Could you check a few things on this model? Use its own coordinates, in mm. A direction names the side the tool comes from. Coordinates: 2 decimals unless noted, no trailing zeros. Loops run counter-clockwise (first coordinate to the right, second up) from the corner with the lowest first, then second, coordinate; pieces in that order, holes last. Notation, with made-up numbers: (78.5, 44.5) -> (121.5, 44.5) arc R8 ccw to (121.5, 51.5) -> close; hole circle Ø5 at (58.25, -30.75). An arc over 180 degrees is marked (long way). One line per question, with ' | ' between items. Start each with the question number.
(1) I'm going to push flat-ended pins straight in: pin 1 Ø6 at (x, y) = (-2, 3.5) entering from -Z; pin 2 Ø1 at (x, y) = (-1, 11.5) entering from -Z; pin 3 Ø4 at (y, z) = (-2.5, -2) entering from -X. Where does each tip first touch, or does it pass through?
(2) Suppose I cut it at C-C (z = 0). Give the number of separate pieces and of enclosed holes in the cut face, plus the area to 3 significant figures.
(3) If we mould it in two halves opening along X, with no side actions, what happens to faces 1 (the face through (-2.3, -6, 0)), 2 (the face through (2.5, -3, 0)), 3 (the face through (0, 0, 0)), 4 (the face through (2.1, -3, 0))? For each: pulls with the +X half, pulls with the -X half, needs draft (parallel to the pull), parting line crosses it, or undercut.
(4) If I drill on line 1 along X through (y, z) = (-0.5, 1); line 2 along X through (y, z) = (6, 0); line 3 along Y through (x, z) = (2.4, 0), over which ranges is the centre line in solid material (lowest first)?
(5) Suppose I cut it at A-A (y = -4.7). Please give me the cut outline in (x, z).
(6) Suppose I cut it at B-B (y = 15.5). Please give me the cut outline in (x, z).
(7) Which directions (+Z, -Z, +X, -X, +Y, -Y) give clear straight access to the entire face, cutting with the end or side of a thin tool? Please do faces 5 (the face through (-2.5, -3, 0)), 6 (the face through (-1.049, 11.693, 4.725)), 7 (the face through (-2.303, -5.268, 0.295)), 8 (the face through (-2.1, -3, 0)).
```python
from build123d import *

# Parameters (mm, degrees)
CONG_1_R                = 0.2
CONG_2_R                = 0.2
CHANFREIN1_SIZE         = 0.7
CHANFREIN1_SIZE2        = 0.454585315
CONG_3_R                = 2
ESQUISSE2_W             = 0.4
ESQUISSE2_H             = 2.6
BOSS_EXTRU_1_DEPTH      = 6
ESQUISSE3_R             = 0.64
ENL_V_MAT_EXTRU_1_DEPTH = 6
CONG_4_R                = 1


with BuildPart() as part:
    # Esquisse1 → Révolution1 (revolve)
    with BuildSketch(Plane.XY):
        with BuildLine():
            Line((0, 18.8), (0, 0))
            Line((0, 0), (3.69, 0))
            Line((3.69, 0), (3.69, 7))
            Line((3.69, 7), (4.84, 7))
            Line((4.84, 7), (4.84, 15))
            Line((4.84, 15), (6.01, 15))
            Line((6.01, 15), (6.01, 16))
            ThreePointArc((6.01, 16), (5.013982948, 16.330092875), (4, 16.6))
            Line((4, 16.6), (4, 15.013190638))
            Line((4, 15.013190638), (3.89, 15.013190638))
            Line((3.89, 15.013190638), (3.89, 18.2))
            ThreePointArc((3.89, 18.2), (1.968000254, 18.649118314), (0, 18.8))
        make_face()
    revolve(axis=Axis((0, 0, 0), (0, 1, 0)))

    # Congé1
    cong_1_edges = [part.edges().sort_by_distance(p)[0] for p in [
        (-3.89, 18.2, 0),
    ]]
    fillet(cong_1_edges, radius=CONG_1_R)

    # Congé2
    cong_2_edges = [part.edges().sort_by_distance(p)[0] for p in [
        (-6.01, 16, 0),
    ]]
    fillet(cong_2_edges, radius=CONG_2_R)

    # Chanfrein1
    chanfrein1_edges = [part.edges().sort_by_distance(p)[0] for p in [
        (-4.84, 7, 0),
    ]]
    chanfrein1_side = [part.faces().sort_by_distance(p)[0] for p in [
        (-4.84, 11, 0),
    ]]
    chamfer(chanfrein1_edges, length=CHANFREIN1_SIZE, length2=CHANFREIN1_SIZE2, reference=chanfrein1_side[0])

    # Congé3
    cong_3_edges = [part.edges().sort_by_distance(p)[0] for p in [
        (-4.84, 7.7, 0),
    ]]
    fillet(cong_3_edges, radius=CONG_3_R)

    # Esquisse2 → Boss.-Extru.1 (add)
    with BuildSketch(Plane.XZ):
        with Locations((2.3, 0)):
            Rectangle(ESQUISSE2_W, ESQUISSE2_H)
        with Locations((-2.3, 0)):
            Rectangle(ESQUISSE2_W, ESQUISSE2_H)
    extrude(amount=BOSS_EXTRU_1_DEPTH)

    # Esquisse3 → Enlèv. mat.-Extru.1 (cut)
    with BuildSketch(Plane.ZY.offset(2.5)):
        with Locations((0, -4.7)):
            Circle(ESQUISSE3_R)
        with BuildLine():
            Line((-1.3, -0.8), (-4.192462756, -0.8))
            Line((-4.192462756, -0.8), (-4.192462756, -7.475627282))
            Line((-4.192462756, -7.475627282), (5.572809524, -7.57510374))
            Line((5.572809524, -7.57510374), (5.225347222, -0.8))
            Line((5.225347222, -0.8), (1.3, -0.8))
            ThreePointArc((1.3, -0.8), (0.901580438, -2.499750503), (1.207561262, -4.218548238))
            ThreePointArc((1.207561262, -4.218548238), (0, -6), (-1.207561262, -4.218548238))
            ThreePointArc((-1.207561262, -4.218548238), (-0.901580438, -2.499750503), (-1.3, -0.8))
        make_face()
    extrude(amount=-ENL_V_MAT_EXTRU_1_DEPTH, mode=Mode.SUBTRACT)

    # Congé4
    cong_4_edges = [part.edges().sort_by_distance(p)[0] for p in [
        (-2.3, -0.8, -1.3),
        (2.3, -0.8, -1.3),
        (2.3, -0.8, 1.3),
        (-2.3, -0.8, 1.3),
    ]]
    fillet(cong_4_edges, radius=CONG_4_R)


solid = part.part
```
Checks:
1) pin 1: stops at z = -3.69 | pin 2: stops at z = -4.81 | pin 3: stops at x = -2.5
2) separate pieces: 3 | enclosed holes: 0 | area: 166 mm^2
3) face 1: needs draft | face 2: pulls with the +X half | face 3: undercut | face 4: undercut
4) line 1: x = -2.5 to -2.1, 2.1 to 2.5 | line 2: x = -3.69 to 3.69 | line 3: y = -6 to -5.34, -4.06 to 18.57
5) outline: (-2.5, -1.3) -> (-2.1, -1.3) -> (-2.1, -0.64) -> (-2.5, -0.64) -> close; (-2.5, 0.64) -> (-2.1, 0.64) -> (-2.1, 1.3) -> (-2.5, 1.3) -> close; (2.1, -1.3) -> (2.5, -1.3) -> (2.5, -0.64) -> (2.1, -0.64) -> close; (2.1, 0.64) -> (2.5, 0.64) -> (2.5, 1.3) -> (2.1, 1.3) -> close
6) outline: circle Ø12.02 at (0, 0); circle Ø7.78 at (0, 0); hole circle Ø8 at (0, 0)
7) face 5: +Z, -Z, -X, -Y | face 6: -Y | face 7: +X, -X | face 8: +Z, -Z, -Y
